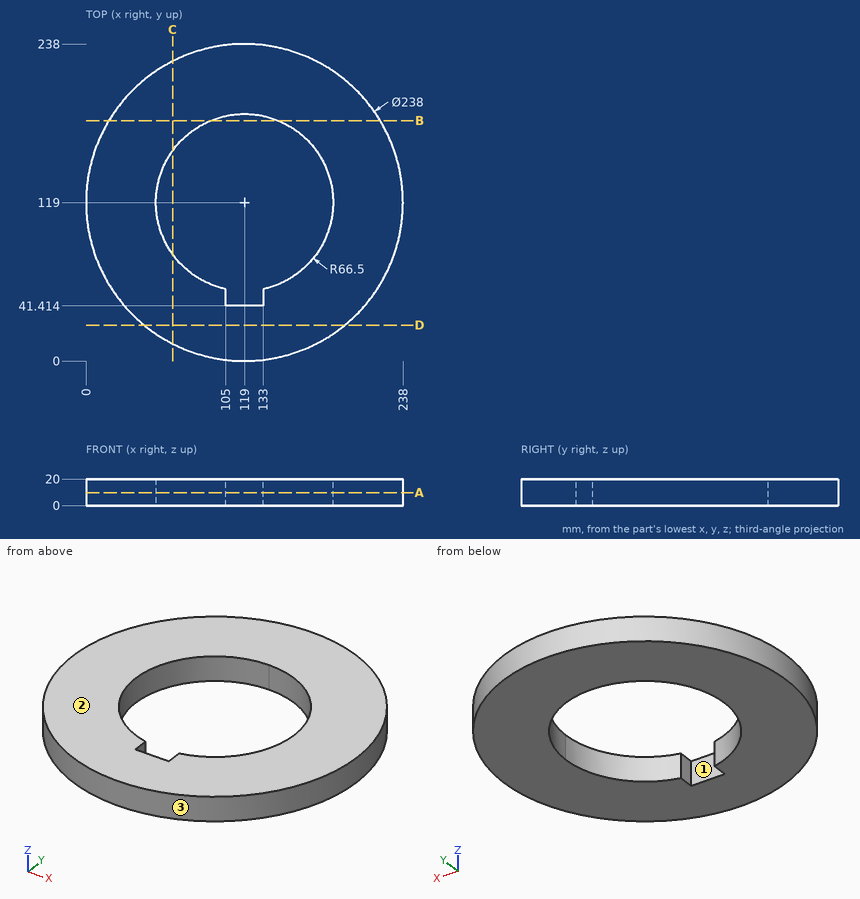
Job drawing, mm, ordinate dimensions from the low corner. One solid piece. Round coordinates to 2 decimals unless told otherwise and drop trailing zeros. Order: outer loops, then holes, each group sorted by start corner. A loop starts at its lowest first (then second) coordinate and runs counter-clockwise, first axis right, second up. Notation, with made-up numbers: M -36.75,48.5 L -13.75,48.5 A29 ccw -13.75,86.5 Z; hole C 74,-25 d11. An arc over 180 degrees is marked long. Write each question's results on one line, items separated by ' | '. Start each with the question number.
(1) Saw through at B-B, the plane y = 180.5. Give the cut face in (x, z), then the cut area to 3 significant figures.
(2) Probe probe 1 along Y at (x, z) = (103, 8); probe 2 along Y at (x, z) = (175, 7.5) (1 decimal); probe 3 along X at (y, z) = (95, 18.5) (1 decimal). List the from-to ranges inside material, lowest first. Write a range as from..to.
(3) Two-plate mould, pull along Y, no slides. Class the marked faces 1, 2 and 3: pulls with the +Y half, pulls with the -Y half, needs draft (parallel to the pull), parting line crosses it, or undercut.
(4) Drop flat-ended pins along their axis: pin 1 (8 mm diameter, centred on x = 112, z = 7, fed in from -Y); pin 2 (5 mm diameter, centred on x = 66.5, z = 3, fed in from +Y); pin 3 (1 mm diameter, centred on y = 52, z = 11.5, fed in from +X) (1 decimal); pin 4 (10 mm diameter, centred on x = 78.5, y = 205.5, fed in from -Z). Give the stop position or say it passes through.
(5) Saw through at A-A, the plane z = 9.75. Give the cut face in (x, y), then the cut area to 3 significant figures.
(6) Saw through at C-C, the plane x = 65. Give the cut face in (y, z), then the cut area to 3 significant figures.
(7) Saw through at D-D, the plane y = 27. Give the cut face in (x, z).
Established:
1) outline: M 17.12,0 L 93.7,0 L 93.7,20 L 17.12,20 Z; M 144.3,0 L 220.88,0 L 220.88,20 L 144.3,20 Z | area: 3,060 mm^2
2) probe 1: y = 1.08..54.45, 183.55..236.92 | probe 2: y = 14..83.1, 154.9..224 | probe 3: x = 2.4..57, 181..235.6
3) face 1: undercut | face 2: needs draft | face 3: parting line crosses it
4) pin 1: stops at y = 0.04 | pin 2: stops at y = 226.99 | pin 3: stops at x = 217.7 | pin 4: stops at z = 0
5) outline: C 119,119 d238; hole M 105,41.41 L 133,41.41 L 133,53.99 A66.5 ccw 185.5,119 A66.5 ccw long 105,53.99 Z | area: 30,300 mm^2
6) outline: M 12.96,0 L 80.19,0 L 80.19,20 L 12.96,20 Z; M 157.81,0 L 225.04,0 L 225.04,20 L 157.81,20 Z | area: 2,690 mm^2
7) outline: M 43.52,0 L 194.48,0 L 194.48,20 L 43.52,20 Z
